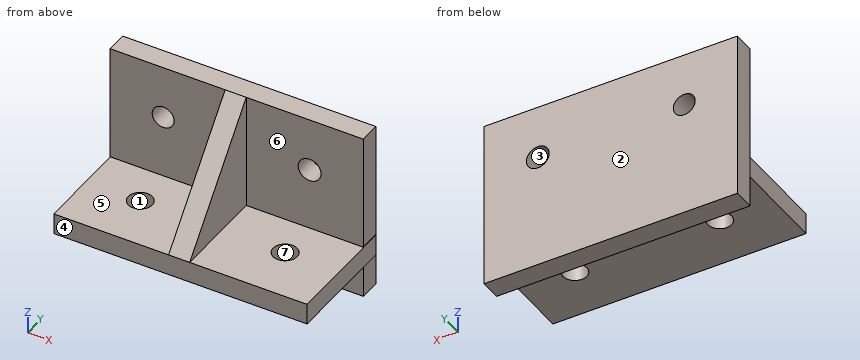
```python
from build123d import *

# Parameters (mm, degrees)
F0_W     = 120
F0_H     = 80
F0_R     = 5.19491
F0_R_2   = 5.424314
F1_DEPTH = 10
F2_W     = 120
F2_H     = 10
F3_DEPTH = 55
F4_R     = 5.684537
F4_R_2   = 5.694204
F5_DEPTH = 10
F6_W     = 10
F6_H     = 45
F7_DEPTH = 55
F9_DEPTH = 25


with BuildPart() as f1:
    # F0 (on Front) → F1 (new body)
    with BuildSketch(Plane.XZ):
        Rectangle(F0_W, F0_H)
        with Locations((-34.80509, 14.80509)):
            Circle(F0_R, mode=Mode.SUBTRACT)
        with Locations((34.575686, 14.575686)):
            Circle(F0_R_2, mode=Mode.SUBTRACT)
    extrude(amount=F1_DEPTH)

    # F2 (on Front) → F3 (join)
    with BuildSketch(Plane.XZ):
        with Locations((0.167052, -20)):
            Rectangle(F2_W, F2_H)
    extrude(amount=F3_DEPTH)

    # F4 (on face) → F5 (cut)
    with BuildSketch(Plane.XY.offset(-15)):
        with Locations((-34.148411, -29.315463)):
            Circle(F4_R)
        with Locations((34.472848, -29.305796)):
            Circle(F4_R_2)
    extrude(amount=-F5_DEPTH, mode=Mode.SUBTRACT)

    # F6 (on face) → F7 (join)
    with BuildSketch(Plane.XY.offset(-15)):
        with Locations((-0.443549, -32.5)):
            Rectangle(F6_W, F6_H)
    extrude(amount=F7_DEPTH)

    # F8 (on face) → F9 (cut)
    with BuildSketch(Plane.YZ.offset(4.556451)):
        Polygon((-55, -15), (-10, 40), (-55, 40), align=None)
    extrude(amount=-F9_DEPTH, mode=Mode.SUBTRACT)


solid = f1.part
```
Check sheet for the modelled part. Datum: model origin and axes. Units: mm. Face numbers are marked on the shaded views. A direction names the side the tool comes from. Round coordinates to 2 decimals unless told otherwise and drop trailing zeros. Write each loop counter-clockwise with the first axis right and the second up, starting at its lowest first coordinate (ties: lowest second). Pieces come first, ordered by that corner, then holes. Notation, with made-up numbers: M -13,-13.5 L 34,-13.5 A17 ccw 34,6.5 Z; hole C -36.75,54.25 d5. An arc over 180 degrees is marked long. Write item = value, one per line. Start each with the question number.
1. Section check D-D, the plane z = -31. Record the cut outline in (x, y), then the cut area to 3 significant figures.
2. Release check for a two-part mould opening along Y. For the marked faces 1, 2, 3 and 4 record: pulls with the +Y half, pulls with the -Y half, needs draft (parallel to the pull), parting line crosses it, or undercut.
3. Section check A-A, the plane z = -9.5. Record the cut outline in (x, y), then the cut area to 4 significant figures.
4. Section check C-C, the plane y = -32.5. Record the cut outline in (x, z), then the cut area to 3 significant figures.
5. Gauge pin test, flat ends, axial feed: pin 1 (8.5 mm diameter, centred on x = 34.58, z = 14.58, fed in from +Y); pin 2 (8 mm diameter, centred on y = -5, z = 10, fed in from +X); pin 3 (12 mm diameter, centred on x = -48, y = -33, fed in from +Z); pin 4 (4 mm diameter, centred on x = 1, y = -38.5, fed in from -Z). Record the tip position at first contact, or that the pin passes through.
6. Scan lines: line 1 (X direction, y = -21, z = -10); line 2 (Z direction, x = -27, y = -16.5); line 3 (Y direction, x = -13.5, z = 22). Record each from-to range of solid material in increasing order. Write a range as [from, to].
7. Tool access check on the marked faces 5, 6 and 7. Record the directions out of +Z, -Z, +X, -X, +Y, -Y that give a thin tool (end or side, any length) a straight path to the whole face; none if there is none.
8. Section check B-B, the plane x = -48. Record the cut outline in (y, z).
Results found:
q1.outline = M -60,-10 L 60,-10 L 60,0 L -60,0 Z
q1.area = 1,200 mm^2
q2.face_1 = undercut
q2.face_2 = pulls with the +Y half
q2.face_3 = needs draft
q2.face_4 = pulls with the -Y half
q3.outline = M -60,-10 L -5.44,-10 L -5.44,-50.5 L 4.56,-50.5 L 4.56,-10 L 60,-10 L 60,0 L -60,0 Z
q3.area = 1,605 mm^2
q4.outline = M -59.83,-25 L -38.86,-25 L -38.86,-15 L -59.83,-15 Z; M -29.44,-25 L 29.76,-25 L 29.76,-15 L 4.56,-15 L 4.56,12.5 L -5.44,12.5 L -5.44,-15 L -29.44,-15 Z; M 39.19,-25 L 60.17,-25 L 60.17,-15 L 39.19,-15 Z
q4.area = 1,290 mm^2
q5.pin_1 = through
q5.pin_2 = 60
q5.pin_3 = -15
q5.pin_4 = -25
q6.line_1 = [-5.44, 4.56]
q6.line_2 = [-25, -15]
q6.line_3 = [-10, 0]
q7.face_5 = +Z, -X, -Y
q7.face_6 = +Z, +X, -Y
q7.face_7 = +Z, -Z
q8.outline = M -55,-25 L -10,-25 L -10,-40 L 0,-40 L 0,40 L -10,40 L -10,-15 L -55,-15 Z
